from build123d import *

# Parameters (mm, degrees)
SKETCH4_W           = 125
SKETCH4_H           = 70
BOSS_EXTRUDE1_DEPTH = 10


with BuildPart() as part:
    # Sketch4 → Boss-Extrude1 (new body)
    with BuildSketch(Plane.XY):
        Polygon((0, 0), (-345, 0), (-366.148351929, 140), (-366.148351929, 170), (-345, 310), (0, 310), (53.851648071, 170), (53.851648071, 140), align=None)
        with BuildLine():
            Line((-262.5, 267.5), (-82.5, 267.5))
            ThreePointArc((-82.5, 267.5), (-65, 250), (-82.5, 232.5))
            Line((-82.5, 232.5), (-262.5, 232.5))
            ThreePointArc((-262.5, 232.5), (-280, 250), (-262.5, 267.5))
        make_face(mode=Mode.SUBTRACT)
        with Locations((-262.5, 95)):
            Rectangle(SKETCH4_W, SKETCH4_H, mode=Mode.SUBTRACT)
        with Locations((-82.5, 95)):
            Rectangle(SKETCH4_W, SKETCH4_H, mode=Mode.SUBTRACT)
    extrude(amount=BOSS_EXTRUDE1_DEPTH)


solid = part.part
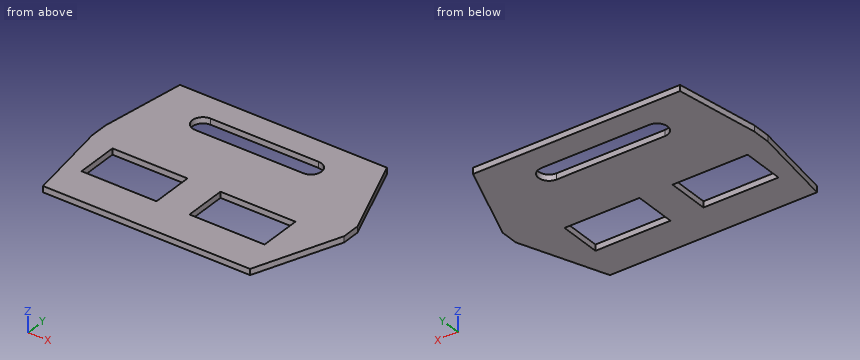
Geometry check sheet. Reference: the model listing, model coordinates, mm. Round coordinates to 2 decimals unless told otherwise and drop trailing zeros. Order: outer loops, then holes, each group sorted by start corner. A loop starts at its lowest first (then second) coordinate and runs counter-clockwise, first axis right, second up. Notation, with made-up numbers: M 73.25,-39.75 L 132.25,-39.75 A15 ccw 132.25,-10.75 Z; hole C 54.5,79 d2. An arc over 180 degrees is marked long. Write each question's results on one line, items separated by ' | '. Start each with the question number.
1. Cross-section at C-C on y = 239. Record the boundary of the cut face in (x, z).
2. Cross-section at D-D on y = 95.5. Record the boundary of the cut face in (x, z), plus the area to 3 significant figures.
3. Cross-section at A-A on x = -168. Record the boundary of the cut face in (y, z), plus the area to 3 significant figures.
4. Cross-section at B-B on z = 4.25. Record the boundary of the cut face in (x, y).
5. Material ranges on L1, parallel to Y at x = -214, z = 7.5; L2, parallel to Y at x = -187, z = 6.5; L3, parallel to X at y = 61.5, z = 4.25, recorded low to high. Write a range as from..to.
Resolved:
1) outline: M -355.73,0 L -276.11,0 L -276.11,10 L -355.73,10 Z; M -68.89,0 L 27.31,0 L 27.31,10 L -68.89,10 Z
2) outline: M -359.43,0 L -325,0 L -325,10 L -359.43,10 Z; M -200,0 L -145,0 L -145,10 L -200,10 Z; M -20,0 L 36.73,0 L 36.73,10 L -20,10 Z | area: 1,460 mm2
3) outline: M 0,0 L 232.5,0 L 232.5,10 L 0,10 Z; M 267.5,0 L 310,0 L 310,10 L 267.5,10 Z | area: 2,750 mm2
4) outline: M -366.15,140 L -345,0 L 0,0 L 53.85,140 L 53.85,170 L 0,310 L -345,310 L -366.15,170 Z; hole M -325,60 L -200,60 L -200,130 L -325,130 Z; hole M -262.5,232.5 L -82.5,232.5 A17.5 ccw -82.5,267.5 L -262.5,267.5 A17.5 ccw Z; hole M -145,60 L -20,60 L -20,130 L -145,130 Z
5) L1: 0..60, 130..232.5, 267.5..310 | L2: 0..232.5, 267.5..310 | L3: -354.29..-325, -200..-145, -20..23.66
